Design review of the part built by this model. Coordinates are the model's own, in mm. Face numbers are marked on the shaded views. A direction names the side the tool comes from. Give positions to 0.01 mm unless a question says otherwise; leave off trailing zeros. Loops run counter-clockwise (first coordinate to the right, second up) from the corner with the lowest first, then second, coordinate; pieces in that order, holes last.
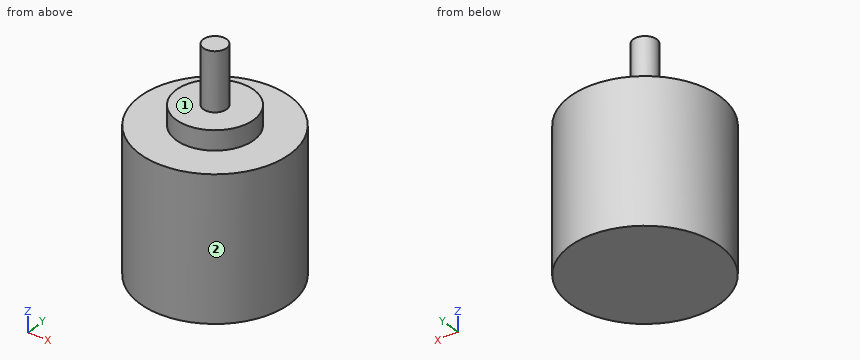
from build123d import *

# Parameters (mm, degrees)
SKETCH1_R           = 19.3
BOSS_EXTRUDE1_DEPTH = 36.7
SKETCH3_R           = 10
BOSS_EXTRUDE2_DEPTH = 5
SKETCH4_R           = 3
BOSS_EXTRUDE3_DEPTH = 15


with BuildPart() as part:
    # Sketch1 → Boss-Extrude1 (new body)
    with BuildSketch(Plane.XY):
        with Locations((-14.127422454, 5.37928778)):
            Circle(SKETCH1_R)
    extrude(amount=BOSS_EXTRUDE1_DEPTH)

    # Sketch3 → Boss-Extrude2 (add)
    with BuildSketch(Plane.XY.offset(36.7)):
        with Locations((-14.127422454, 5.37928778)):
            Circle(SKETCH3_R)
    extrude(amount=BOSS_EXTRUDE2_DEPTH)

    # Sketch4 → Boss-Extrude3 (add)
    with BuildSketch(Plane.XY.offset(41.7)):
        with Locations((-14.127422454, 5.37928778)):
            Circle(SKETCH4_R)
    extrude(amount=BOSS_EXTRUDE3_DEPTH)


solid = part.part
Q1. Insertion check: pin 1 (3 mm diameter, centred on y = 1, z = 40, fed in from +X); pin 2 (1 mm diameter, centred on x = -26.5, z = 28.5, fed in from -Y); pin 3 (4 mm diameter, centred on x = -2.5, z = 7, fed in from +Y). Each pin has a flat end and moves straight along its axis. Give the tip position at first contact, or say it passes through.
Results:
pin 1: stops at x = -4.55
pin 2: stops at y = -9.84
pin 3: stops at y = 22.11
Q2. Take a section at B-B (y = -3). Give the boundary of the cut face in (x, z).
Results:
outline: (-31.51, 0) - (3.26, 0) - (3.26, 36.7) - (-8.67, 36.7) - (-8.67, 41.7) - (-19.59, 41.7) - (-19.59, 36.7) - (-31.51, 36.7) - close
Q3. Wall thickness on line 1 (Z direction, x = -29, y = 2.5); line 2 (Z direction, x = -8.5, y = -2.5); line 3 (X direction, y = 6, z = 6): over which ranges is each line inside the solid? List them lowest first.
Results:
line 1: z = 0 to 36.7
line 2: z = 0 to 41.7
line 3: x = -33.42 to 5.16
Q4. Take a section at D-D (x = -18). Give the boundary of the cut face in (y, z), plus the area to 3 significant figures.
Results:
outline: (-13.53, 0) - (24.29, 0) - (24.29, 36.7) - (14.6, 36.7) - (14.6, 41.7) - (-3.84, 41.7) - (-3.84, 36.7) - (-13.53, 36.7) - close
area: 1,480 mm2
Q5. Take a section at A-A (x = -13). Give the boundary of the cut face in (y, z), plus the area to 3 significant figures.
Results:
outline: (-13.89, 0) - (24.65, 0) - (24.65, 36.7) - (15.32, 36.7) - (15.32, 41.7) - (8.16, 41.7) - (8.16, 56.7) - (2.6, 56.7) - (2.6, 41.7) - (-4.56, 41.7) - (-4.56, 36.7) - (-13.89, 36.7) - close
area: 1,600 mm2
Q6. Tool access review of the marked faces 1 and 2: name each direction out of +Z, -Z, +X, -X, +Y, -Y from which nothing blocks a thin tool from reaching the whole face with its end or side.
Results:
face 1: +Z
face 2: +Z, -Z
Q7. Take a section at C-C (z = 31). Give the boundary of the cut face in (x, y), plus the area to 3 significant figures.
Results:
outline: circle Ø38.6 at (-14.13, 5.38)
area: 1,170 mm2
